from build123d import *

# Parameters (mm, degrees)
SKETCH1_W           = 375
SKETCH1_H           = 240
SKETCH1_R           = 5.181490122
SKETCH1_R_2         = 6.018247546
SKETCH1_R_3         = 6.106953205
SKETCH1_R_4         = 3.5
SKETCH1_R_5         = 6.35
BOSS_EXTRUDE1_DEPTH = 6.35


with BuildPart() as part:
    # Sketch1 → Boss-Extrude1 (new body)
    with BuildSketch(Plane(origin=(0, 0, 0), x_dir=(1, 0, 0), z_dir=(0, 1, 0))):
        with Locations((187.5, -120)):
            Rectangle(SKETCH1_W, SKETCH1_H)
        with Locations(Location((15, -15, 0), (0, 0, 270))):
            Circle(SKETCH1_R, mode=Mode.SUBTRACT)
        with Locations(Location((39.680379951, -15, 0), (0, 0, 270))):
            Circle(SKETCH1_R, mode=Mode.SUBTRACT)
        with Locations(Location((25, -225, 0), (0, 0, 270))):
            Circle(SKETCH1_R, mode=Mode.SUBTRACT)
        with Locations(Location((70, -225, 0), (0, 0, 270))):
            Circle(SKETCH1_R, mode=Mode.SUBTRACT)
        with Locations(Location((193.34, -225, 0), (0, 0, 270))):
            Circle(SKETCH1_R_2, mode=Mode.SUBTRACT)
        with Locations(Location((257.244291662, -225, 0), (0, 0, 270))):
            Circle(SKETCH1_R_3, mode=Mode.SUBTRACT)
        with Locations(Location((41.566569972, -43, 0), (0, 0, 270))):
            Circle(SKETCH1_R_4, mode=Mode.SUBTRACT)
        with Locations(Location((41.566569972, -197, 0), (0, 0, 270))):
            Circle(SKETCH1_R_4, mode=Mode.SUBTRACT)
        with Locations(Location((330.566569972, -197, 0), (0, 0, 270))):
            Circle(SKETCH1_R_4, mode=Mode.SUBTRACT)
        with Locations(Location((330.566569972, -43, 0), (0, 0, 270))):
            Circle(SKETCH1_R_4, mode=Mode.SUBTRACT)
        with Locations(Location((209.82, -20, 0), (0, 0, 270))):
            Circle(SKETCH1_R_5, mode=Mode.SUBTRACT)
        with Locations(Location((123.622084245, -20, 0), (0, 0, 270))):
            Circle(SKETCH1_R_5, mode=Mode.SUBTRACT)
        with Locations(Location((296.017915755, -20, 0), (0, 0, 270))):
            Circle(SKETCH1_R_5, mode=Mode.SUBTRACT)
    extrude(amount=-BOSS_EXTRUDE1_DEPTH)


solid = part.part
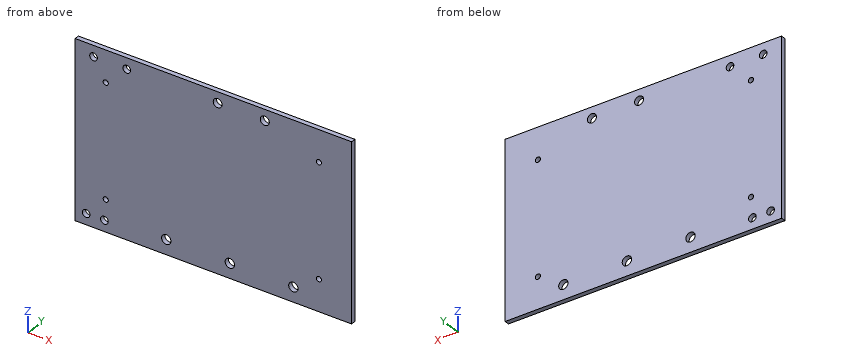
Work out the finished part from the listing and answer in its coordinate system (mm). Coordinates: 2 decimals unless noted, no trailing zeros. Write each loop counter-clockwise with the first axis right and the second up, starting at its lowest first coordinate (ties: lowest second). Pieces come first, ordered by that corner, then holes. Notation, with made-up numbers: (57.5, 57) - (111.5, 57) arc R26 ccw to (111.5, 83) - close; hole circle Ø3 at (-38.75, 35.5). An arc over 180 degrees is marked (long way). One line per question, with ' | ' between items.
1) Find section B-B, the plane x = 209.82. Determine the outline of the cut face in (y, z), and give its area (3 significant figures).
Checks:
outline: (-6.35, 0) - (0, 0) - (0, 13.65) - (-6.35, 13.65) - close; (-6.35, 26.35) - (0, 26.35) - (0, 240) - (-6.35, 240) - close | area: 1,440 mm2
2) Consider probe 1 along X at (y, z) = (-2, 225); probe 2 along X at (y, z) = (-2.5, 197); probe 3 along X at (y, z) = (-2.25, 224). Determine where each line is inside the solid, lowest interval first. Write a range as [from, to].
Checks:
probe 1: [0, 19.82], [30.18, 64.82], [75.18, 187.32], [199.36, 251.14], [263.35, 375] | probe 2: [0, 38.07], [45.07, 327.07], [334.07, 375] | probe 3: [0, 19.92], [30.08, 64.92], [75.08, 187.41], [199.27, 251.22], [263.27, 375]
3) A flat-ended cylindrical pin translates along its axis: P1, Ø16.5, axis at x = 123.62, z = 20, coming from the -Y side. Find the tip coordinate at first contact, or state that the pin passes through.
Checks:
P1: y = -6.35
4) Find section A-A, the plane x = 15. Determine the outline of the cut face in (y, z), and give its area (3 significant figures).
Checks:
outline: (-6.35, 0) - (0, 0) - (0, 9.82) - (-6.35, 9.82) - close; (-6.35, 20.18) - (0, 20.18) - (0, 240) - (-6.35, 240) - close | area: 1,460 mm2
